Solid Edge part; units mm, degrees
sketch "Sketch1" plane through (0, 0, 0) normal (0, 0, 1) x (1, 0, 0)
  circle A0 centre (0, 0) radius 1.5
extrude "Protrusion1" add sketch "Sketch1" along normal blind 16
sketch "Sketch2" plane through (0, 0, 16) normal (0, 0, 1) x (1, 0, 0)
  circle A0 centre (0, 0) radius 2.25
extrude "ProtrusiónExtruida_2" add sketch "Sketch2" along normal blind 1.5
sketch "Sketch3" plane through (0, 0, 17.5) normal (0, 0, 1) x (1, 0, 0)
  line L0 (0, 1.402) -> (1.2141, 0.701)
  line L1 (1.2141, 0.701) -> (1.2141, -0.701)
  line L2 (1.2141, -0.701) -> (0, -1.402)
  line L3 (0, -1.402) -> (-1.2141, -0.701)
  line L4 (-1.2141, -0.701) -> (-1.2141, 0.701)
  line L5 (-1.2141, 0.701) -> (0, 1.402)
extrude "VaciadoExtruido_1" cut sketch "Sketch3" against normal blind 1
chamfer "Chaflán_1" distance 0.4 angle 45 1 edges at (-1.5, 0, 0)
properties material "Acero inoxidable, 303"
Verification items for the finished model (mm, model axes). A direction names the side the tool comes from. Round coordinates to 2 decimals unless told otherwise and drop trailing zeros. Order: outer loops, then holes, each group sorted by start corner. A loop starts at its lowest first (then second) coordinate and runs counter-clockwise, first axis right, second up. Notation, with made-up numbers: (52.5, -7) - (100.5, -7) arc R30 ccw to (100.5, 29) - close; hole circle Ø3 at (-18, 11.5). An arc over 180 degrees is marked (long way). Use CSV: the item, a comma, the result in double quotes. Start each with the question number.
1) Section check B-B, the plane z = 4.5. Record the cut outline in (x, y), plus the area to 3 significant figures.
2) Thickness scan on L1, parallel to Z at x = 0.55, y = -2; L2, parallel to X at y = -0.1, z = 13.5; L3, parallel to Z at x = -0.85, y = -0.35. Record the ranges inside material, lowest first.
3) Mould release check, pull along Y, two halves, no side actions. Record for faces 4 (the cylindrical face through (-1.5, -0.07, 8.09)), 5 (the flat face through (1, -1, 17.5)), 6 (the flat face through (0.616, -1.047, 17.007)): +Y half, -Y half, draft (parallel to the pull), parting line (faces both ways), or undercut.
4) Section check A-A, the plane y = 0. Record the cut outline in (x, z).
5) Go/stop test with flat-tipped pins: P1, Ø0.8, axis at y = 0.5, z = 17, coming from the +X side; P2, Ø1.5, axis at x = 0.5, z = 12.5, coming from the +Y side; P3, Ø1.5, axis at y = 2, z = 13, coming from the -X side. Record where each tip stops, or that it passes through.
6) Access from +Z, -Z, +X, -X, +Y, -Y to the whole of each face (thin tool, end or side, straight path). Record for faces 1 (the flat face through (-2, 0, 16)), 2 (the flat face through (-0.599, -1.056, 17.007)), 3 (the cylindrical face through (-0.29, -2.23, 16.74)).
7) Section check C-C, the plane x = -1.65. Record the cut outline in (y, z).
Answers:
1,outline,"circle Ø3 at (0, 0)"
1,area,"7.07 mm²"
2,L1,"z = 16 to 17.5"
2,L2,"x = -1.5 to 1.5"
2,L3,"z = 0 to 16.5"
3,face 4,"parting line"
3,face 5,"draft"
3,face 6,"undercut"
4,outline,"(-2.25, 16) - (-1.5, 16) - (-1.5, 0.4) - (-1.1, 0) - (1.1, 0) - (1.5, 0.4) - (1.5, 16) - (2.25, 16) - (2.25, 17.5) - (1.21, 17.5) - (1.21, 16.5) - (-1.21, 16.5) - (-1.21, 17.5) - (-2.25, 17.5) - close"
5,P1,"stops at x = 2.25"
5,P2,"stops at y = 1.5"
5,P3,"stops at x = -0.83"
6,face 1,"-Z"
6,face 2,"+Z"
6,face 3,"+Z, -Z"
7,outline,"(-1.53, 16) - (1.53, 16) - (1.53, 17.5) - (-1.53, 17.5) - close"
